Source: three-view drawing plus pictorial views. Frame: mm from the lowest corner of the part. A direction names the side the tool comes from. Round coordinates to 2 decimals unless told otherwise and drop trailing zeros. Order: outer loops, then holes, each group sorted by start corner. A loop starts at its lowest first (then second) coordinate and runs counter-clockwise, first axis right, second up. Notation, with made-up numbers: (27.5, -8.75) - (84.5, -8.75) arc R12 ccw to (84.5, 9.25) - close; hole circle Ø10 at (27.25, 40). An arc over 180 degrees is marked (long way). One line per item, written item: value. Start each with the question number.
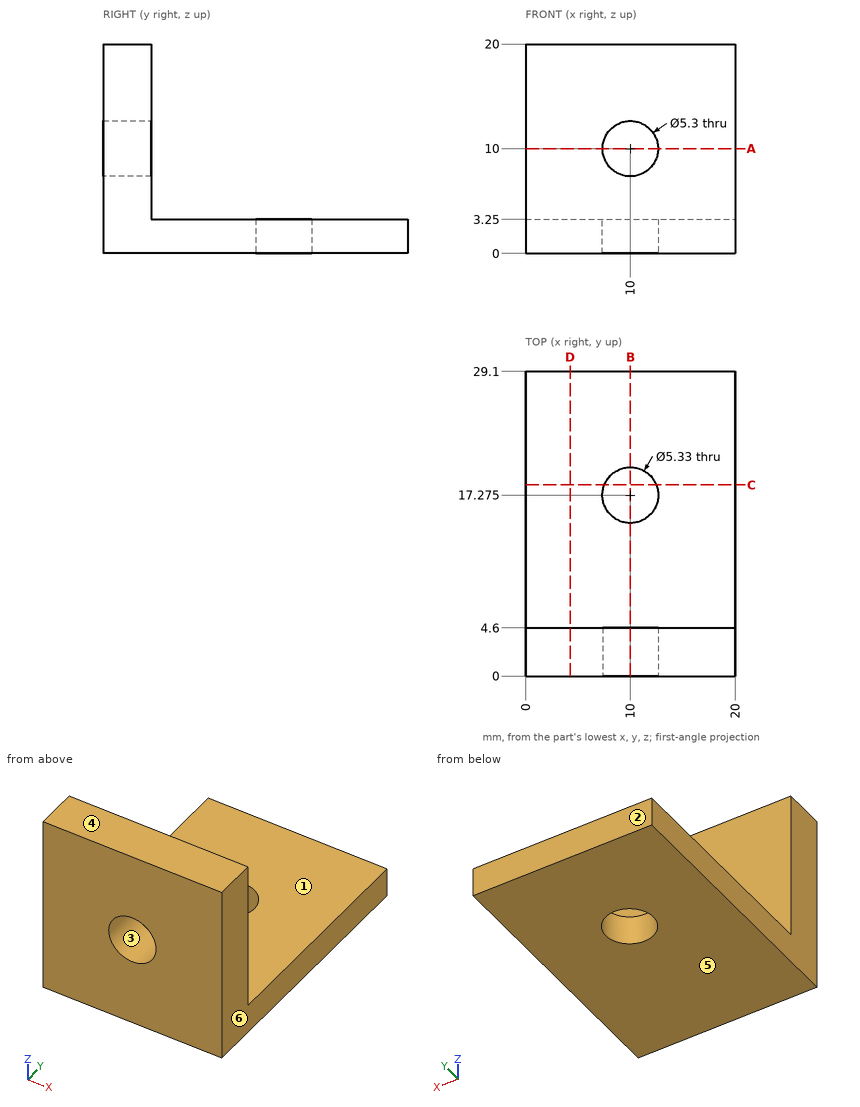
Item 1: Section query B-B on x = 10. Return loops of the section in (y, z), and give its area (3 significant figures).
Item 2: Line query: L1, parallel to X at y = 1.3, z = 10; L2, parallel to Z at x = 13, y = 23.5; L3, parallel to Y at x = 2, z = 10.25. Output: solid intervals per line, ascending.
Item 3: Reachability of the marked faces 1 and 2 from +Z, -Z, +X, -X, +Y, -Y: full face, straight path, thin tool, end or side. Return the list, or none.
Item 4: Section query D-D on x = 4.25. Return loops of the section in (y, z).
Item 5: First-contact query: pin 1 Ø10 at (x, y) = (8, 24) entering from +Z; pin 2 Ø6 at (x, z) = (3.5, 14.5) entering from +Y. Flat tips, straight axial feed; report the tip coordinate or a pass-through.
Item 6: Section query C-C on y = 18.25. Return loops of the section in (x, z), and give its area (3 significant figures).
Item 7: Pull-direction query (Z, two-part tool) for the marked faces 3, 4, 5 and 6; classes: released by +Z, released by -Z, zero draft, split by the parting line, or undercut.
Item 8: Section query A-A on z = 10. Return loops of the section in (x, y), and give its area (3 significant figures).
Geometry results:
1. outline: (0, 0) - (14.61, 0) - (14.61, 3.25) - (4.6, 3.25) - (4.6, 7.35) - (0, 7.35) - close; (0, 12.65) - (4.6, 12.65) - (4.6, 20) - (0, 20) - close; (19.94, 0) - (29.1, 0) - (29.1, 3.25) - (19.94, 3.25) - close
1. area: 130 mm^2
2. L1: x = 0 to 7.35, 12.65 to 20
2. L2: z = 0 to 3.25
2. L3: y = 0 to 4.6
3. face 1: +Z, +X, -X, +Y
3. face 2: +Z, -Z, +X, -X, +Y
4. outline: (0, 0) - (29.1, 0) - (29.1, 3.25) - (4.6, 3.25) - (4.6, 20) - (0, 20) - close
5. pin 1: stops at z = 3.25
5. pin 2: stops at y = 4.6
6. outline: (0, 0) - (7.52, 0) - (7.52, 3.25) - (0, 3.25) - close; (12.48, 0) - (20, 0) - (20, 3.25) - (12.48, 3.25) - close
6. area: 48.9 mm^2
7. face 3: undercut
7. face 4: released by +Z
7. face 5: released by -Z
7. face 6: zero draft
8. outline: (0, 0) - (7.35, 0) - (7.35, 4.6) - (0, 4.6) - close; (12.65, 0) - (20, 0) - (20, 4.6) - (12.65, 4.6) - close
8. area: 67.6 mm^2
